Autodesk Inventor part; units mm, degrees
ref_plane "YZ Plane" through (0, 0, 0) normal (1, 0, 0) x (0, 1, 0)
ref_plane "XZ Plane" through (0, 0, 0) normal (0, 1, 0) x (-1, 0, 0)
ref_plane "XY Plane" through (0, 0, 0) normal (0, 0, 1) x (1, 0, 0)
sketch "スケッチ1" plane through (0, 0, 0) normal (0, 0, 1) x (1, 0, 0)
  circle A0 centre (0, 0) radius 46
  circle A1 centre (0, 0) radius 50
  circle A2 centre (0, 0) radius 42
  line L0 (0, 0) -> (0, 54.8528)
  line L1 (0, 0) -> (-20.7697, 50.1426)
  circle A3 centre (-17.6034, 42.4985) radius 1.5
  circle A4 centre (-42.4985, 17.6034) radius 1.5
  circle A5 centre (-42.4985, -17.6034) radius 1.5
  circle A6 centre (-17.6034, -42.4985) radius 1.5
  circle A7 centre (17.6034, -42.4985) radius 1.5
  circle A8 centre (42.4985, -17.6034) radius 1.5
  circle A9 centre (42.4985, 17.6034) radius 1.5
  circle A10 centre (17.6034, 42.4985) radius 1.5
  line L2 (0, 0) -> (-55.1659, -46.2897)
  line L3 (-55.1659, -46.2897) -> (-55.1659, 46.2897)
  line L4 (-55.1659, 46.2897) -> (0, 0)
  line L5 (0, 0) -> (-76.7662, 0)
  point P0 (-32.1739, -26.9971)
  point P1 (-32.1739, 26.9971)
  point P2 (-38.3022, 32.1394)
  point P3 (-38.3022, -32.1394)
  dimension "d0" = 92
  dimension "d1" = 100
  dimension "d2" = 84
  dimension "d3" = 22.5
  dimension "d4" = 3
  dimension "d7" = 360
  dimension "d9" = 80
  dimension "d10" = 40
extrude "押し出し1" add sketch "スケッチ1" along normal blind 8 contours L2 A1 L5 A0 A5 | A0 A5 L5 A2 L2 | A2 L5 A0 A4 L4 | L4 A0 A4 L5 A1
fillet "フィレット1" radius 4 4 edges at (-32.1739, -26.9971, 4) (-38.3022, -32.1394, 4) (-38.3022, 32.1394, 4) (-32.1739, 26.9971, 4)
sketch "スケッチ2" plane through (0, 0, 8) normal (0, 0, 1) x (1, 0, 0)
  circle A0 centre (-42.4985, -17.6034) radius 1.5
  circle A1 centre (-42.4985, -17.6034) radius 3
  circle A2 centre (-42.4985, 17.6034) radius 1.5
  circle A3 centre (-42.4985, 17.6034) radius 3
  point P0 (0, 0)
  dimension "d14" = 6
  dimension "d15" = 6
extrude "押し出し2" cut sketch "スケッチ2" against normal blind 3 contours A0 | A1 | A2 | A3
equation "\"d10\" = 0.5 * d9"
properties part number "legparts_10"
Verification items for the finished model (mm, model axes). A direction names the side the tool comes from. Coordinates: 2 decimals unless noted, no trailing zeros. Order: outer loops, then holes, each group sorted by start corner. A loop starts at its lowest first (then second) coordinate and runs counter-clockwise, first axis right, second up. Notation, with made-up numbers: (21, -36.75) - (32, -36.75) arc R18 cw to (32, -18.75) - close; hole circle Ø7 at (-21, 61). An arc over 180 degrees is marked (long way). Return JSON: item names as keys, results as strings.
(1) Section check D-D, the plane x = -48. Record the cut outline in (y, z), and give its area (3 significant figures).
Filled sheet:
{"outline": "(-14, 0) - (14, 0) - (14, 8) - (-14, 8) - close", "area": "224 mm^2"}
(2) Thickness scan on line 1 along Y through (x, z) = (-44, 6.5); line 2 along Y through (x, z) = (-36, 2.5); line 3 along X through (y, z) = (0.5, 4). Record the ranges inside material, lowest first.
Filled sheet:
{"line 1": "y = -23.75 to -20.2, -15.01 to 15.01, 20.2 to 23.75", "line 2": "y = -30.02 to -21.63, 21.63 to 30.02", "line 3": "x = -50 to -42"}
(3) Mould release check, pull along X, two halves, no side actions. Record for faces 3 (the cylindrical face through (-42.694, 16.116, 2.465)), 4 (the cylindrical face through (-38.243, -30.352, 4.056)), 5 (the flat face through (-44, 0, 8)), 6 (the cylindrical face through (-33.704, 26.873, 4.056)): pulls with the +X half, pulls with the -X half, needs draft (parallel to the pull), parting line crosses it, or undercut.
Filled sheet:
{"face 3": "undercut", "face 4": "parting line crosses it", "face 5": "needs draft", "face 6": "pulls with the +X half"}
(4) Section check B-B, the plane x = -38.5. Record the cut outline in (y, z).
Filled sheet:
{"outline": "(-30.31, 0) - (-16.79, 0) - (-16.79, 8) - (-30.31, 8) - close; (16.79, 0) - (30.31, 0) - (30.31, 8) - (16.79, 8) - close"}
(5) Section check A-A, the plane z = 2.75. Give the number of separate pieces and of enclosed holes in the cut face, and give its area (3 significant figures).
Filled sheet:
{"separate pieces": "1", "enclosed holes": "2", "area": "486 mm^2"}
(6) Go/stop test with flat-tipped pins: pin 1 (3.5 mm diameter, centred on x = -42.5, y = -17.6, fed in from +Z); pin 2 (2.5 mm diameter, centred on x = -42.5, y = 17.6, fed in from -Z); pin 3 (3 mm diameter, centred on y = -9.5, z = 1, fed in from +X); pin 4 (4 mm diameter, centred on x = -47, z = 3.5, fed in from +Y). Record where each tip stops, or that it passes through.
Filled sheet:
{"pin 1": "stops at z = 5", "pin 2": "passes through", "pin 3": "stops at x = -40.53", "pin 4": "stops at y = 21.79"}
(7) Access from +Z, -Z, +X, -X, +Y, -Y to the whole of each face (thin tool, end or side, straight path). Record for faces 1 (the cylindrical face through (-45.496, 17.735, 6.521)), 2 (the cylindrical face through (-42.82, -16.14, 2.46)).
Filled sheet:
{"face 1": "+Z", "face 2": "+Z, -Z"}
(8) Section check C-C, the plane y = -17. Record the cut outline in (x, z).
Filled sheet:
{"outline": "(-47.02, 0) - (-43.87, 0) - (-43.87, 5) - (-45.44, 5) - (-45.44, 8) - (-47.02, 8) - close; (-41.13, 0) - (-38.41, 0) - (-38.41, 8) - (-39.56, 8) - (-39.56, 5) - (-41.13, 5) - close"}
